Source: CAD feature listing. Evaluate the final solid. Frame: model axes, mm. Give positions to 0.01 mm unless a question says otherwise; leave off trailing zeros. Order: outer loops, then holes, each group sorted by start corner. A loop starts at its lowest first (then second) coordinate and runs counter-clockwise, first axis right, second up. Notation, with made-up numbers: M -24,21 L 9,21 A31 ccw 9,49 Z; hole C 43.25,16 d5. An arc over 180 degrees is marked long. Answer in a Markdown table with one row per item. Add a question column.
(1) Section query C-C, the plane z = 28. Return loops of the section in (x, y), plus the area to 3 significant figures.
(2) Section query D-D, the plane z = 43.5. Return loops of the section in (x, y).
(3) Pin query (flat end, axial travel): P1, Ø1.5, axis at x = -0.5, z = 33.5, coming from the -Y side; P2, Ø1, axis at y = 1, z = 24.5, coming from the -X side; P3, Ø1, axis at x = 0.5, z = 11.5, coming from the -Y side. Return the tip coordinate at first contact, or that it passes through.
(4) Mould query, pull axis Z, two halves, no side actions, for faces 1 (the face through (-0.367, -1.654, 30.031)), 2 (the face through (0, 0, 0)), 3 (the face through (-1.11, -0.85, 2.46)). Classes: pulls with the +Z half, pulls with the -Z half, needs draft (parallel to the pull), parting line crosses it, or undercut.
(5) Section query A-A, the plane x = 0. Return loops of the section in (y, z).
(6) Material intervals for line 1 along Y through (x, z) = (0.1, 38); line 2 along Z through (x, y) = (-0.1, 0.7); line 3 along X through (y, z) = (0.6, 15), sorted ascending.
from build123d import *

# Parameters (mm, degrees)
F0_R     = 1.397
F1_DEPTH = 5
F2_R     = 2.349867992
F3_DEPTH = 50.8
F3_TAPER = 1.5


with BuildPart() as f1:
    # F0 (on Top) → F1 (new body)
    with BuildSketch(Plane.XY):
        Circle(F0_R)
    extrude(amount=F1_DEPTH)

    # F2 (on face) → F3 (join)
    with BuildSketch(Plane.XY.offset(5)):
        Circle(F2_R)
    extrude(amount=F3_DEPTH, taper=F3_TAPER)

    # F4 (on face) → F5 (revolve)
    with BuildSketch(Plane.XY.offset(55.8)):
        with BuildLine():
            Line((0, -1.778), (0, 1.778))
            ThreePointArc((0, 1.778), (-1.778, 0), (0, -1.778))
        make_face()
    revolve(axis=Axis((0, 0, 55.8), (0, -1, 0)))


solid = f1.part
Values follow:
| question | item | result |
|---|---|---|
| 1 | outline | C 0,0 d3.5 |
| 1 | area | 9.59 mm² |
| 2 | outline | C 0,0 d2.68 |
| 3 | P1 | stops at y = -1.62 |
| 3 | P2 | stops at x = -1.77 |
| 3 | P3 | stops at y = -2.19 |
| 4 | face 1 | undercut |
| 4 | face 2 | pulls with the -Z half |
| 4 | face 3 | needs draft |
| 5 | outline | M -2.35,5 L -1.4,5 L -1.4,0 L 1.4,0 L 1.4,5 L 2.35,5 L 1.06,54.37 A1.78 ccw long -1.06,54.37 Z |
| 6 | line 1 | y = -1.48 to 1.48 |
| 6 | line 2 | z = 0 to 57.43 |
| 6 | line 3 | x = -2 to 2 |
